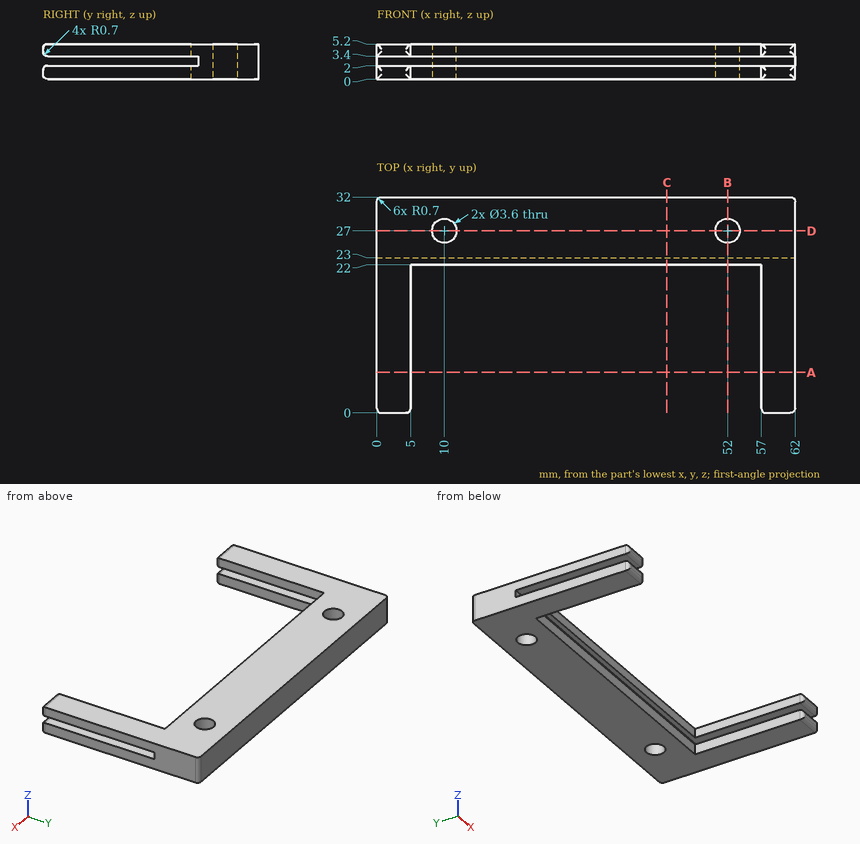
For this review, use the dimensioned drawing (mm, ordinates from the lowest corner) and the shaded views. Coordinates: 2 decimals unless noted, no trailing zeros. Loops run counter-clockwise (first coordinate to the right, second up) from the corner with the lowest first, then second, coordinate; pieces in that order, holes last. Notation, with made-up numbers: (20.5, 49) -> (25.5, 49) arc R28 cw to (25.5, 68) -> close; hole circle Ø7 at (34, 55). An arc over 180 degrees is marked (long way). Return JSON: item names as keys, results as strings. Group by question number.
(1) For pin 1 Ø0.9 at (x, z) = (22, 4.5) entering from -Y; pin 2 Ø6 at (x, y) = (19.5, 16.5) entering from -Z; pin 3 Ø18 at (x, y) = (26.5, 16) entering from +Z, all flat-tipped, find the tip position at first contact; note any pin that passes through.
(2) Consider section B-B, the plane x = 52. Give the boundary of the cut face in (y, z), plus the area to 3 significant figures.
(3) To check wall thickness, follow L1, parallel to X at y = 27, z = 2.8; L2, parallel to Y at x = 52, z = 2.1; L3, parallel to Z at x = 58, y = 9. State the ranges of each line that lie inside material, in increasing order.
(4) Consider section A-A, the plane y = 6. Give the boundary of the cut face in (x, z).
(5) Consider section C-C, the plane x = 43. Give the boundary of the cut face in (y, z), plus the area to 3 significant figures.
(6) Consider section D-D, the plane y = 27. Give the boundary of the cut face in (x, z), plus the area to 3 significant figures.
Results below:
{
 "1": {"pin 1": "stops at y = 22", "pin 2": "passes through", "pin 3": "stops at z = 5.2"},
 "2": {"outline": "(22, 0) -> (25.2, 0) -> (25.2, 5.2) -> (22, 5.2) -> (22, 3.4) -> (23, 3.4) -> (23, 2) -> (22, 2) -> close; (28.8, 0) -> (32, 0) -> (32, 5.2) -> (28.8, 5.2) -> close", "area": "31.9 mm2"},
 "3": {"L1": "x = 0 to 8.2, 11.8 to 50.2, 53.8 to 62", "L2": "y = 23 to 25.2, 28.8 to 32", "L3": "z = 0 to 2, 3.4 to 5.2"},
 "4": {"outline": "(0, 0) -> (5, 0) -> (5, 2) -> (0, 2) -> close; (0, 3.4) -> (5, 3.4) -> (5, 5.2) -> (0, 5.2) -> close; (57, 0) -> (62, 0) -> (62, 2) -> (57, 2) -> close; (57, 3.4) -> (62, 3.4) -> (62, 5.2) -> (57, 5.2) -> close"},
 "5": {"outline": "(22, 0) -> (32, 0) -> (32, 5.2) -> (22, 5.2) -> (22, 3.4) -> (23, 3.4) -> (23, 2) -> (22, 2) -> close", "area": "50.6 mm2"},
 "6": {"outline": "(0, 0) -> (8.2, 0) -> (8.2, 5.2) -> (0, 5.2) -> close; (11.8, 0) -> (50.2, 0) -> (50.2, 5.2) -> (11.8, 5.2) -> close; (53.8, 0) -> (62, 0) -> (62, 5.2) -> (53.8, 5.2) -> close", "area": "285 mm2"}
}
